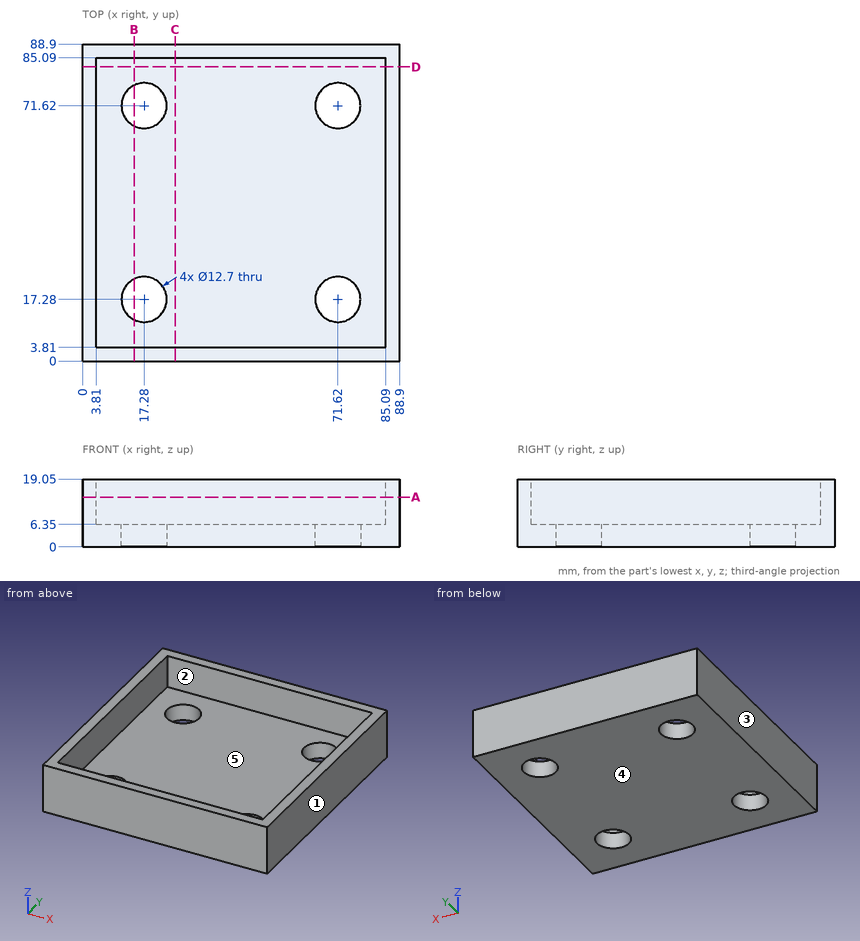
Can you work these out from the drawing? Everything is in mm from the part's minimum corner. A direction names the side the tool comes from. Round coordinates to 2 decimals unless told otherwise and drop trailing zeros. Loops run counter-clockwise (first coordinate to the right, second up) from the corner with the lowest first, then second, coordinate; pieces in that order, holes last. Notation, with made-up numbers: (-13.5, 16.25) - (22.5, 16.25) arc R37 ccw to (22.5, 53.25) - close; hole circle Ø10 at (31.25, 84). An arc over 180 degrees is marked (long way). One line per question, with ' | ' between items. Start each with the question number.
Q1. Please list where these lines run through material, in increasing order: line 1 (X direction, y = 42, z = 13.25); line 2 (X direction, y = 66, z = 1.5) (1 decimal). Write a range as [from, to].
Q2. I want a section at C-C (x = 26). Write out the boundary of the cut face in (y, z).
Q3. We'd pull the mould along X, two halves only. Please class the marked faces 1, 2 and 3: +X half, -X half, draft (parallel to the pull), parting line (faces both ways), or undercut.
Q4. Will this pin go through, and if not, where does the flat tip stop? pin 1 (24.5 mm diameter, centred on x = 47, y = 64, fed in from +Z).
Q5. I want a section at A-A (z = 14). Write out the boundary of the cut face in (x, y).
Q6. I want a section at B-B (x = 14.5). Write out the boundary of the cut face in (y, z), then the cut area to 3 significant figures.
Q7. For the marked faces 4 and 5, which set-ups out of +Z, -Z, +X, -X, +Y, -Y let a thin tool reach every point of the face, with its end or its side?
Response values:
1) line 1: x = [0, 3.81], [85.09, 88.9] | line 2: x = [0, 14.3], [20.2, 68.7], [74.6, 88.9]
2) outline: (0, 0) - (88.9, 0) - (88.9, 19.05) - (85.09, 19.05) - (85.09, 6.35) - (3.81, 6.35) - (3.81, 19.05) - (0, 19.05) - close
3) face 1: +X half | face 2: undercut | face 3: -X half
4) pin 1: stops at z = 6.35
5) outline: (0, 0) - (88.9, 0) - (88.9, 88.9) - (0, 88.9) - close; hole (3.81, 3.81) - (85.09, 3.81) - (85.09, 85.09) - (3.81, 85.09) - close
6) outline: (0, 0) - (11.57, 0) - (11.57, 6.35) - (3.81, 6.35) - (3.81, 19.05) - (0, 19.05) - close; (22.99, 0) - (65.91, 0) - (65.91, 6.35) - (22.99, 6.35) - close; (77.33, 0) - (88.9, 0) - (88.9, 19.05) - (85.09, 19.05) - (85.09, 6.35) - (77.33, 6.35) - close | area: 516 mm²
7) face 4: -Z, +X, -X, +Y, -Y | face 5: +Z
